Source: CAD feature listing. Evaluate the final solid. Frame: model axes, mm. A direction names the side the tool comes from. Give positions to 0.01 mm unless a question says otherwise; leave off trailing zeros. Loops run counter-clockwise (first coordinate to the right, second up) from the corner with the lowest first, then second, coordinate; pieces in that order, holes last. Notation, with made-up numbers: M -33.5,-39 L 5.5,-39 A15 cw 5.5,-12 Z; hole C 28.25,6 d9. An arc over 180 degrees is marked long. Put each result on its own line as item: value.
from build123d import *

# Parameters (mm, degrees)
EXTRUDE_1_DEPTH = 2
EXTRUDE_3_DEPTH = 0.5
FILLET_1_R      = 1
EXTRUDE_4_DEPTH = 1
EXTRUDE_5_DEPTH = 2


with BuildPart() as part:
    # 스케치1 → 보스-돌출1 (new body)
    with BuildSketch(Plane.XY):
        Polygon((3, 16), (0, 13), (0, 3), (3, 0), (47, 0), (50, 3), (50, 13), (47, 16), align=None)
    extrude(amount=EXTRUDE_1_DEPTH)

    # 스케치3 → 보스-돌출3 (add)
    with BuildSketch(Plane(origin=(0, 0, 0), x_dir=(-1, 0, 0), z_dir=(0, 0, -1))):
        Polygon((0, 13), (-3, 16), (-22, 16), (-22, 0), (-3, 0), (0, 3), align=None)
    extrude(amount=EXTRUDE_3_DEPTH)

    # 필렛1
    fillet_1_edges = [part.edges().sort_by_distance(p)[0] for p in [
        (0, 8, -0.5),
    ]]
    fillet(fillet_1_edges, radius=FILLET_1_R)

    # 스케치2 → 보스-돌출4 (add)
    with BuildSketch(Plane(origin=(0, 0, 0), x_dir=(-1, 0, 0), z_dir=(0, 0, -1))):
        Polygon((-47, 0), (-40, 0), (-40, 16), (-47, 16), (-50, 13), (-50, 3), align=None)
    extrude(amount=EXTRUDE_4_DEPTH)

    # 스케치4 → 보스-돌출5 (add)
    with BuildSketch(Plane(origin=(0, 0, -1), x_dir=(-1, 0, 0), z_dir=(0, 0, -1))):
        Polygon((-46, 12.618802154), (-50, 10.309401077), (-50, 5.690598923), (-46, 3.381197846), (-42, 5.690598923), (-42, 10.309401077), align=None)
    extrude(amount=EXTRUDE_5_DEPTH)


solid = part.part
1. Section query D-D (z = -1.65). Output: boundary loops of the cut face in (x, y), plus the area to 3 significant figures.
Found:
outline: M 42,5.69 L 46,3.38 L 50,5.69 L 50,10.31 L 46,12.62 L 42,10.31 Z
area: 55.4 mm^2
2. Material intervals for line 1 (Z direction, x = 11.5, y = 2.75); line 2 (X direction, y = 8.25, z = -0.05); line 3 (Z direction, x = 26, y = 6), sorted ascending. Write a range as from..to.
Found:
line 1: -0.5..2
line 2: 0.16..22, 40..50
line 3: 0..2
3. Section query B-B (y = 8.25). Output: boundary loops of the cut face in (x, z).
Found:
outline: M 0,0.5 A1 ccw 1,-0.5 L 22,-0.5 L 22,0 L 40,0 L 40,-1 L 42,-1 L 42,-3 L 50,-3 L 50,2 L 0,2 Z
4. Access query for faces 1 (the flat face through (48.028, 4.552, -1.986)), 2 (the flat face through (43.972, 11.448, -1.986)), 3 (the flat face through (40, 7.9, -0.5)), 4 (the flat face through (12, 8, -0.5)), 5 (the flat face through (2, 1, 1)). Directions: +Z, -Z, +X, -X, +Y, -Y. A direction counts if a zero-diameter tool reaches every point of the face in a straight line with its end or side. Return the directions, or none.
Found:
face 1: -Z, +X, -Y
face 2: -Z, -X, +Y
face 3: -Z, +Y, -Y
face 4: -Z, -X, +Y, -Y
face 5: +Z, -Z, -X, -Y
5. Section query C-C (x = 34.5). Output: boundary loops of the cut face in (y, z), plus the area to 3 significant figures.
Found:
outline: M 0,0 L 16,0 L 16,2 L 0,2 Z
area: 32.0 mm^2
6. Contact query for flat-ended pins moving along their axis: P1, Ø1.5, axis at x = 42.5, y = 11, coming from the -Z side; P2, Ø1.5, axis at x = 29, y = 3, coming from the -Z side; P3, Ø0.6, axis at y = 8.5, z = -2, coming from the -X side; P4, Ø8, axis at x = 10.5, y = 9.5, coming from the -Z side. Output: stop coordinate, or through.
Found:
P1: z = -3
P2: z = 0
P3: x = 42
P4: z = -0.5
7. Section query A-A (z = 1.4). Output: boundary loops of the cut face in (x, y), plus the area to 3 significant figures.
Found:
outline: M 0,3 L 3,0 L 47,0 L 50,3 L 50,13 L 47,16 L 3,16 L 0,13 Z
area: 782 mm^2
